```python
from build123d import *

# Parameters (mm, degrees)
CROQUIS1_W              = 20
CROQUIS1_H              = 20
SALIENTE_EXTRUIR1_DEPTH = 5
CROQUIS2_W              = 5
CROQUIS2_H              = 10
SALIENTE_EXTRUIR2_DEPTH = 20
SALIENTE_EXTRUIR3_REACH = 32.822
CROQUIS3_R              = 2.5
REDONDEO4_R             = 1


with BuildPart() as part:
    # Croquis1 → Saliente-Extruir1 (new body)
    with BuildSketch(Plane(origin=(0, 0, 0), x_dir=(1, 0, 0), z_dir=(0, 1, 0))):
        Rectangle(CROQUIS1_W, CROQUIS1_H)
    extrude(amount=SALIENTE_EXTRUIR1_DEPTH)

    # Croquis2 → Saliente-Extruir2 (add)
    with BuildSketch(Plane(origin=(0, 5, 0), x_dir=(1, 0, 0), z_dir=(0, 1, 0))):
        with Locations((-7.5, 0)):
            Rectangle(CROQUIS2_W, CROQUIS2_H)
        with Locations((7.5, 0)):
            Rectangle(CROQUIS2_W, CROQUIS2_H)
    extrude(amount=SALIENTE_EXTRUIR2_DEPTH)

    # Croquis3 → Saliente-Extruir3 (add, up to next)
    with BuildSketch(Plane.ZY.offset(-5), mode=Mode.PRIVATE) as saliente_extruir3_sk1:
        with Locations(Location((0, 20, 0), (0, 0, 180))):
            Circle(CROQUIS3_R)
    saliente_extruir3_tool1 = extrude(saliente_extruir3_sk1.sketch, amount=SALIENTE_EXTRUIR3_REACH, mode=Mode.PRIVATE) - part.part
    add(saliente_extruir3_tool1.solids().sort_by_distance((5, 20, 0))[0])

    # Redondeo4
    redondeo4_edges = [part.edges().sort_by_distance(p)[0] for p in [
        (10, 5, 7.5),
        (0, 5, -10),
        (-10, 5, 7.5),
        (-10, 15, -5),
        (-7.5, 5, 5),
        (-10, 15, 5),
        (-5, 5, 0),
        (-5, 15, 5),
        (-7.5, 5, -5),
        (-5, 15, -5),
        (-10, 25, 0),
        (-7.5, 25, 5),
        (-5, 25, 0),
        (-7.5, 25, -5),
        (10, 5, -7.5),
        (5, 5, 0),
        (5, 15, -5),
        (7.5, 5, 5),
        (5, 15, 5),
        (10, 15, 5),
        (7.5, 5, -5),
        (10, 15, -5),
        (5, 25, 0),
        (7.5, 25, 5),
        (10, 25, 0),
        (7.5, 25, -5),
        (-10, 5, -7.5),
        (0, 0, -10),
        (10, 0, 0),
        (0, 0, 10),
        (-10, 0, 0),
        (0, 5, 10),
        (-10, 2.5, -10),
        (10, 2.5, -10),
        (10, 2.5, 10),
        (-10, 2.5, 10),
    ]]
    fillet(redondeo4_edges, radius=REDONDEO4_R)


solid = part.part
```
Here's how the part is built. I have some questions about the finished solid (model axes, mm). A direction names the side the tool comes from. Coordinates: 2 decimals unless noted, no trailing zeros. Order: outer loops, then holes, each group sorted by start corner. A loop starts at its lowest first (then second) coordinate and runs counter-clockwise, first axis right, second up. Notation, with made-up numbers: (-37, -2) -> (-25, -2) arc R25 cw to (-25, 36) -> close; hole circle Ø1 at (82, -32). An arc over 180 degrees is marked (long way). Return JSON: item names as keys, results as strings.
1) On a 3-axis mill with a long thin cutter (end or side, diameter ignored), from which of +Z, -Z, +X, -X, +Y, -Y can I reach the whole of each face in a straight line? I mean faces 1 (the cylindrical face through (5.285, 24.699, -0.056)), 2 (the cylindrical face through (-5.301, 15.126, 4.715)), 3 (the cylindrical face through (-9.715, 4.699, -7.521)). Say none if no direction works.
Conclusion:
{"face 1": "+Z, -Z, +Y", "face 2": "+Z, +Y", "face 3": "-Z, -X, +Y"}
2) If we section it at B-B on z = 2: List the corners of the cut face in (x, y) for me, plus the area to 3 significant figures.
Conclusion:
{"outline": "(-10, 1) arc R1 ccw to (-9, 0) -> (9, 0) arc R1 ccw to (10, 1) -> (10, 24) arc R1 ccw to (9, 25) -> (6, 25) arc R1 ccw to (5, 24) -> (5, 21.5) -> (-5, 21.5) -> (-5, 24) arc R1 ccw to (-6, 25) -> (-9, 25) arc R1 ccw to (-10, 24) -> close; hole (-5, 6) arc R1 ccw to (-4, 5) -> (4, 5) arc R1 ccw to (5, 6) -> (5, 18.5) -> (-5, 18.5) -> close", "area": "329 mm²"}
3) If we section it at D-D on z = -8.5: List the corners of the cut face in (x, y) for me, plus the area to 3 significant figures.
Conclusion:
{"outline": "(-10, 1) arc R1 ccw to (-9, 0) -> (9, 0) arc R1 ccw to (10, 1) -> (10, 4) arc R1 ccw to (9, 5) -> (-9, 5) arc R1 ccw to (-10, 4) -> close", "area": "99.1 mm²"}
4) Thinking about a two-plate mould opening in Y: for faces 4 (the cylindrical face through (9.699, 2.521, 9.715)), 5 (the cylindrical face through (4.699, 5.285, -0.056)), 6 (the cylindrical face through (0.126, 0.301, 9.715)), which applies, +Y half, -Y half, draft (parallel to the pull), parting line (faces both ways), or undercut?
Conclusion:
{"face 4": "draft", "face 5": "undercut", "face 6": "-Y half"}
5) I'm going to push flat-ended pins straight in: P1, Ø6, axis at x = 6.5, y = 18, coming from the +Z side; P2, Ø0.9, axis at x = -7.5, y = 10.5, coming from the -Z side; P3, Ø12, axis at x = 5.5, z = 2, coming from the +Y side. Where does each tip first touch, or does it pass through?
Conclusion:
{"P1": "stops at z = 5", "P2": "stops at z = -5", "P3": "stops at y = 25"}
6) If we section it at C-C on y = 20: List the corners of the cut face in (x, z) for me, plus the area to 3 significant figures.
Conclusion:
{"outline": "(-10, -4) arc R1 ccw to (-9, -5) -> (-6, -5) arc R1 ccw to (-5, -4) -> (-5, -2.5) -> (5, -2.5) -> (5, -4) arc R1 ccw to (6, -5) -> (9, -5) arc R1 ccw to (10, -4) -> (10, 4) arc R1 ccw to (9, 5) -> (6, 5) arc R1 ccw to (5, 4) -> (5, 2.5) -> (-5, 2.5) -> (-5, 4) arc R1 ccw to (-6, 5) -> (-9, 5) arc R1 ccw to (-10, 4) -> close", "area": "148 mm²"}
7) If we section it at A-A on y = 9: List the corners of the cut face in (x, z) for me.
Conclusion:
{"outline": "(-10, -4) arc R1 ccw to (-9, -5) -> (-6, -5) arc R1 ccw to (-5, -4) -> (-5, 4) arc R1 ccw to (-6, 5) -> (-9, 5) arc R1 ccw to (-10, 4) -> close; (5, -4) arc R1 ccw to (6, -5) -> (9, -5) arc R1 ccw to (10, -4) -> (10, 4) arc R1 ccw to (9, 5) -> (6, 5) arc R1 ccw to (5, 4) -> close"}
8) If I drill on probe 1 along X at (y, z) = (11.75, -2.5); probe 2 along Y at (x, z) = (1, -6); probe 3 along Y at (x, z) = (1, 1), over which ranges is the centre line in solid material (lowest first)?
Conclusion:
{"probe 1": "x = -10 to -5, 5 to 10", "probe 2": "y = 0 to 5", "probe 3": "y = 0 to 5, 17.71 to 22.29"}
